Build history of the part. All positions in model axes, mm. A direction names the side the tool comes from. Round coordinates to 2 decimals unless told otherwise and drop trailing zeros. Loops run counter-clockwise (first coordinate to the right, second up) from the corner with the lowest first, then second, coordinate; pieces in that order, holes last. Notation, with made-up numbers: (11.5, 78.25) - (55.5, 78.25) arc R24 cw to (55.5, 103.25) - close; hole circle Ø2 at (41, -37). An arc over 180 degrees is marked (long way). Use a Markdown table: item, result.
from build123d import *

# Parameters (mm, degrees)
F0_W      = 25
F0_H      = 45
F1_DEPTH  = 25
F3_DEPTH  = 25
F5_DEPTH  = 25
F6_W      = 5
F6_H      = 12
F7_DEPTH  = 12
F9_DEPTH  = 25
F10_R     = 5
F11_W     = 5
F11_H     = 12
F12_DEPTH = 12
F14_DEPTH = 25
F15_R     = 5
F16_W     = 19
F16_H     = 6
F17_DEPTH = 19
F19_DEPTH = 12
F20_R     = 5
F21_R     = 5
F22_DEPTH = 2
F24_DEPTH = 25
F27_DEPTH = 4.3
F28_DEPTH = 5
F30_DEPTH = 8


with BuildPart() as f1:
    # F0 (on Front) → F1 (new body)
    with BuildSketch(Plane.XZ):
        with Locations((12.5, 22.5)):
            Rectangle(F0_W, F0_H)
    extrude(amount=F1_DEPTH)

    # F2 (on face) → F3 (cut)
    with BuildSketch(Plane.XZ.offset(25)):
        with BuildLine():
            ThreePointArc((16.5, 37), (9.6715728753, 39.8284271247), (12.5, 33))
            ThreePointArc((12.5, 33), (15.3284271247, 34.1715728753), (16.5, 37))
        make_face()
    extrude(amount=-F3_DEPTH, mode=Mode.SUBTRACT)

    # F4 (on face) → F5 (cut)
    with BuildSketch(Plane(origin=(0, 0, 0), x_dir=(0, -1, 0), z_dir=(-1, 0, 0))):
        with BuildLine():
            ThreePointArc((16.5, 25), (9.6715728753, 27.8284271247), (12.5, 21))
            ThreePointArc((12.5, 21), (15.3284271247, 22.1715728753), (16.5, 25))
        make_face()
    extrude(amount=-F5_DEPTH, mode=Mode.SUBTRACT)

    # F6 (on face) → F7 (join)
    with BuildSketch(Plane(origin=(0, 0, 0), x_dir=(0, -1, 0), z_dir=(-1, 0, 0))):
        with Locations((2.5, 31)):
            Rectangle(F6_W, F6_H)
    extrude(amount=F7_DEPTH)

    # F8 (on face) → F9 (cut)
    with BuildSketch(Plane.XZ.offset(5)):
        with BuildLine():
            ThreePointArc((-6, 33.5), (-8.5, 31), (-6, 28.5))
            Line((-6, 28.5), (-6, 33.5))
        make_face()
        with BuildLine():
            Line((-6, 33.5), (-6, 28.5))
            ThreePointArc((-6, 28.5), (-4.232233047, 29.232233047), (-3.5, 31))
            ThreePointArc((-3.5, 31), (-4.232233047, 32.767766953), (-6, 33.5))
        make_face()
    extrude(amount=-F9_DEPTH, mode=Mode.SUBTRACT)

    # F10
    f10_edges = [f1.edges().sort_by_distance(p)[0] for p in [
        (-12, -2.5, 37),
        (-12, -2.5, 25),
        (0, -2.5, 37),
    ]]
    fillet(f10_edges, radius=F10_R)

    # F11 (on face) → F12 (join)
    with BuildSketch(Plane.XZ.offset(25)):
        with Locations((22.5, 31)):
            Rectangle(F11_W, F11_H)
    extrude(amount=F12_DEPTH)

    # F13 (on face) → F14 (cut)
    with BuildSketch(Plane(origin=(20, 0, 0), x_dir=(0, -1, 0), z_dir=(-1, 0, 0))):
        with BuildLine():
            ThreePointArc((31, 33.5), (28.5, 31), (31, 28.5))
            Line((31, 28.5), (31, 33.5))
        make_face()
        with BuildLine():
            Line((31, 33.5), (31, 28.5))
            ThreePointArc((31, 28.5), (32.767766953, 29.232233047), (33.5, 31))
            ThreePointArc((33.5, 31), (32.767766953, 32.767766953), (31, 33.5))
        make_face()
    extrude(amount=-F14_DEPTH, mode=Mode.SUBTRACT)

    # F15
    f15_edges = [f1.edges().sort_by_distance(p)[0] for p in [
        (22.5, -37, 37),
        (22.5, -37, 25),
        (22.5, -25, 25),
    ]]
    fillet(f15_edges, radius=F15_R)

    # F16 (on face) → F17 (cut)
    with BuildSketch(Plane(origin=(0, 0, 0), x_dir=(0, -1, 0), z_dir=(-1, 0, 0))):
        with Locations((15.5, 7)):
            Rectangle(F16_W, F16_H)
    extrude(amount=-F17_DEPTH, mode=Mode.SUBTRACT)

    # F18 (on face) → F19 (cut)
    with BuildSketch(Plane(origin=(0, 0, 0), x_dir=(1, 0, 0), z_dir=(0, 0, -1))):
        Polygon((17.5, 21.443375673), (17.5, 18.556624327), (20, 17.1132486541), (22.5, 18.556624327), (22.5, 20), (20, 20), (20, 22.8867513459), align=None)
        Polygon((22.5, 21.443375673), (20, 22.8867513459), (20, 20), (22.5, 20), align=None)
    extrude(amount=-F19_DEPTH, mode=Mode.SUBTRACT)

    # F20
    f20_edges = [f1.edges().sort_by_distance(p)[0] for p in [
        (19, -6, 7),
    ]]
    fillet(f20_edges, radius=F20_R)

    # F21
    f21_edges = [f1.edges().sort_by_distance(p)[0] for p in [
        (0, -25, 2),
        (0, -25, 27.5),
    ]]
    fillet(f21_edges, radius=F21_R)

    # F22 (cut): a face of the model
    f22_faces = [f1.faces().sort_by_distance(p)[0] for p in [
        (12.59855993, -12.40144007, 45),
    ]]
    extrude(f22_faces, amount=-F22_DEPTH, mode=Mode.SUBTRACT)

    # F23 (on face) → F24 (cut)
    with BuildSketch(Plane.XZ.offset(25)):
        Polygon((25, 10), (19, 10), (19, 4), (5, 4), (5, 0), (25, 0), align=None)
        Polygon((19, 4), (19, 10), (5, 10), (0, 10), (0, 0), (5, 0), (5, 4), align=None)
    extrude(amount=-F24_DEPTH, mode=Mode.SUBTRACT)

    # F26 (on offset) → F27 (cut)
    with BuildSketch(Plane(origin=(0, 0, 15), x_dir=(1, 0, 0), z_dir=(0, 0, -1))):
        Polygon((24, 17.6905989232), (24, 22.3094010768), (20, 24.6188021535), (16, 22.3094010768), (16, 17.6905989232), (20, 15.3811978465), align=None)
        Polygon((20, 24.6188021535), (24, 22.3094010768), (24, 30.3094010768), (16, 30.3094010768), (16, 22.3094010768), align=None)
    extrude(amount=-F27_DEPTH, mode=Mode.SUBTRACT)

    # F28 (cut): a face of the model
    f28_faces = [f1.faces().sort_by_distance(p)[0] for p in [
        (20, -20, 12),
    ]]
    extrude(f28_faces, amount=-F28_DEPTH, mode=Mode.SUBTRACT)

    # F29 (on face) → F30 (join)
    with BuildSketch(Plane(origin=(0, 0, 10), x_dir=(1, 0, 0), z_dir=(0, 0, -1))):
        with BuildLine():
            ThreePointArc((0, 6), (0.8786796564, 3.8786796564), (3, 3))
            Line((3, 3), (22, 3))
            ThreePointArc((22, 3), (24.1213203436, 3.8786796564), (25, 6))
            ThreePointArc((25, 6), (24.1213203436, 8.1213203436), (22, 9))
            Line((22, 9), (3, 9))
            ThreePointArc((3, 9), (0.8786796564, 8.1213203436), (0, 6))
        make_face()
    extrude(amount=F30_DEPTH)


solid = f1.part
Q1. Cut at B-B, the plane x = 6. List the corners of the cut face in (y, z), plus the area to 3 significant figures.
Results found:
| item | result |
|---|---|
| outline | (-25, 10) - (-9, 10) - (-9, 2) - (-3, 2) - (-3, 10) - (0, 10) - (0, 43) - (-25, 43) - close; hole circle Ø8 at (-12.5, 25) |
| area | 823 mm2 |
Q2. Drop flat-ended pins along their axis: pin 1 (4 mm diameter, centred on y = -18, z = 18.5, fed in from -X); pin 2 (1 mm diameter, centred on x = 16, z = 19, fed in from -Y); pin 3 (9.5 mm diameter, centred on y = -28, z = 30.5, fed in from -X); pin 4 (5 mm diameter, centred on x = 12.5, z = 37, fed in from +Y). Give the stop position or say it passes through.
Results found:
| item | result |
|---|---|
| pin 1 | stops at x = 0 |
| pin 2 | stops at y = -25 |
| pin 3 | stops at x = 1.2 |
| pin 4 | passes through |
Q3. Cut at C-C, the plane y = -14.5. List the corners of the cut face in (x, z), plus the area to 3 significant figures.
Results found:
| item | result |
|---|---|
| outline | (0, 10) - (25, 10) - (25, 21.54) - (0, 21.54) - close; (0, 28.46) - (25, 28.46) - (25, 43) - (0, 43) - close; hole circle Ø8 at (12.5, 37) |
| area | 602 mm2 |
Q4. Probe line 1 (X direction, y = -11.75, z = 37); line 2 (Z direction, x = 10.5, y = -12.5); line 3 (X direction, y = -18.5, z = 18). List the from-to ranges inside material, lowest first.
Results found:
| item | result |
|---|---|
| line 1 | x = 0 to 8.5, 16.5 to 25 |
| line 2 | z = 10 to 21, 29 to 33.54, 40.46 to 43 |
| line 3 | x = 0 to 16, 24 to 25 |
Q5. Pull direction Z, two halves, no side cores. Call faces 5 (the face through (22.5, -20, 12)), 6 (the face through (18, -22, 15)), 7 (the face through (23, -26, 23)): pulls with the +Z half, pulls with the -Z half, needs draft (parallel to the pull), parting line crosses it, or undercut.
Results found:
| item | result |
|---|---|
| face 5 | needs draft |
| face 6 | undercut |
| face 7 | pulls with the -Z half |
Q6. Cut at A-A, the plane z = 13.5. List the corners of the cut face in (x, y), plus the area to 3 significant figures.
Results found:
| item | result |
|---|---|
| outline | (0, -20) arc R5 ccw to (5, -25) - (25, -25) - (25, 0) - (0, 0) - close; hole (17.5, -21.44) - (20, -22.89) - (22.5, -21.44) - (22.5, -18.56) - (20, -17.11) - (17.5, -18.56) - close |
| area | 598 mm2 |
Q7. Which spindle directions (+Z, -Z, +X, -X, +Y, -Y) get a long thin tool onto all of the face, cutting with end or side? Do faces 1 (the face through (-6, -2, 37)), 2 (the face through (17.5, -20, 12)), 3 (the face through (24, -21, 17)), 4 (the face through (-3, -2, 25)). Say none if no direction does.
Results found:
| item | result |
|---|---|
| face 1 | +Z, -X, +Y, -Y |
| face 2 | -Z |
| face 3 | -Y |
| face 4 | -Z, -X, +Y, -Y |
